Design review of the part built by this model. Coordinates are the model's own, in mm. A direction names the side the tool comes from. Coordinates: 2 decimals unless noted, no trailing zeros. Loops run counter-clockwise (first coordinate to the right, second up) from the corner with the lowest first, then second, coordinate; pieces in that order, holes last.
Q1. Draft analysis for pull direction Y (two halves, no side actions). For faces 5 (the face through (2, 55.32, 65)), 6 (the face through (2, 25, -42.5)), 7 (the face through (2, 8, 0)), state which applies: released by +Y, released by -Y, zero draft, split by the parting line, or undercut.
Q2. Add section B-B on x = 4.05. Give the boundary of the cut face in (y, z).
Q3. For P1, Ø1.5, axis at x = 2.5, y = 7, coming from the -Z side; P2, Ø2.5, axis at x = 2.5, y = 124, coming from the +Z side; P3, Ø2.5, axis at x = 3, z = -40.5, coming from the +Y side, all flat-tipped, find the tip position at first contact; note any pin that passes through.
Q4. Add section A-A on z = 12.5. Give the boundary of the cut face in (x, y).
Q5. Machinability: for faces 1 (the face through (2, 12.82, -40)), 2 (the face through (2, 81, -37.5)), 3 (the face through (2, 103, 62.5)), 4 (the face through (2, -72, 0)), which of the approach directions +Z, -Z, +X, -X, +Y, -Y give a long, thin tool a straight path to every point of the face, cutting with its end or side? Answer none if there is none.
Q6. Add section C-C on y = -55.5. Give the boundary of the cut face in (x, z), and give its area (3 significant figures).
Q7. Add section D-D on y = 66.5. Give the boundary of the cut face in (x, z).
Q8. Wall thickness on probe 1 along Z at (x, y) = (1.85, 7); probe 2 along Z at (x, y) = (3.6, 53.5); probe 3 along Z at (x, y) = (2.95, 69.5): over which ranges is each line inside the solid? List them lowest first.
```python
from build123d import *

# Parameters (mm, degrees)
F0_R     = 30
F0_W     = 5
F0_H     = 25
F1_DEPTH = 5


with BuildPart() as f1:
    # F0 (on Right) → F1 (new body)
    with BuildSketch(Plane.YZ):
        Polygon((125.319932, 62.5), (80.319932, 62.5), (80.319932, 67.5), (55.319932, 67.5), (55.319932, 62.5), (10.319932, 62.5), (-74.680068, 62.5), (-74.680068, 25), (-69.680068, 25), (-69.680068, 0), (-74.680068, 0), (-74.680068, -37.5), (12.819932, -37.5), (12.819932, -42.5), (37.819932, -42.5), (37.819932, -37.5), (125.319932, -37.5), (125.319932, 0), (120.319932, 0), (120.319932, 25), (125.319932, 25), align=None)
        with Locations((-32.180068, 12.5)):
            Circle(F0_R, mode=Mode.SUBTRACT)
        with Locations((7.819932, 12.5)):
            Rectangle(F0_W, F0_H, mode=Mode.SUBTRACT)
    extrude(amount=F1_DEPTH)


solid = f1.part
```
Entries:
1. face 5: released by -Y
1. face 6: zero draft
1. face 7: undercut
2. outline: (-74.68, -37.5) - (12.82, -37.5) - (12.82, -42.5) - (37.82, -42.5) - (37.82, -37.5) - (125.32, -37.5) - (125.32, 0) - (120.32, 0) - (120.32, 25) - (125.32, 25) - (125.32, 62.5) - (80.32, 62.5) - (80.32, 67.5) - (55.32, 67.5) - (55.32, 62.5) - (-74.68, 62.5) - (-74.68, 25) - (-69.68, 25) - (-69.68, 0) - (-74.68, 0) - close; hole circle Ø60 at (-32.18, 12.5); hole (5.32, 0) - (10.32, 0) - (10.32, 25) - (5.32, 25) - close
3. P1: stops at z = -37.5
3. P2: stops at z = 62.5
3. P3: stops at y = 37.82
4. outline: (0, -69.68) - (5, -69.68) - (5, -62.18) - (0, -62.18) - close; (0, -2.18) - (5, -2.18) - (5, 5.32) - (0, 5.32) - close; (0, 10.32) - (5, 10.32) - (5, 120.32) - (0, 120.32) - close
5. face 1: -Z, +X, -X, -Y
5. face 2: -Z, +X, -X, +Y
5. face 3: +Z, +X, -X, +Y
5. face 4: +X, -X, -Y
6. outline: (0, -37.5) - (5, -37.5) - (5, -6.37) - (0, -6.37) - close; (0, 31.37) - (5, 31.37) - (5, 62.5) - (0, 62.5) - close
6. area: 311 mm2
7. outline: (0, -37.5) - (5, -37.5) - (5, 67.5) - (0, 67.5) - close
8. probe 1: z = -37.5 to 0, 25 to 62.5
8. probe 2: z = -37.5 to 62.5
8. probe 3: z = -37.5 to 67.5
